from build123d import *

# Parameters (mm, degrees)
F1_DEPTH = 3
F3_DEPTH = 3


with BuildPart() as f1:
    # F0 (on Right) → F1 (new body)
    with BuildSketch(Plane.YZ):
        with BuildLine():
            ThreePointArc((0, -35), (-35, 0), (0, 35))
            Line((0, 35), (0, 50))
            Line((0, 50), (-22, 50))
            ThreePointArc((-22, 50), (-29.119444, 48.689931), (-35.306192, 44.931351))
            Line((-35.306192, 44.931351), (-125, -35))
            Line((-125, -35), (-125, -100))
            Line((-125, -100), (-105, -100))
            Line((-105, -100), (0, -50))
            Line((0, -50), (0, -35))
        make_face()
        with BuildLine():
            ThreePointArc((-96.275498, -75.908841), (-103.504138, -75.479065), (-107, -69.137387))
            Line((-107, -69.137387), (-107, -46.431792))
            ThreePointArc((-107, -46.431792), (-106.343744, -43.363703), (-104.489822, -40.832535))
            Line((-104.489822, -40.832535), (-65.699873, -6.264563))
            ThreePointArc((-65.699873, -6.264563), (-57.267065, -4.57705), (-51.677673, -11.113001))
            ThreePointArc((-51.677673, -11.113001), (-46.996343, -24.335108), (-38.322833, -35.358229))
            ThreePointArc((-38.322833, -35.358229), (-36.281412, -38.203278), (-35.560135, -41.629861))
            ThreePointArc((-35.560135, -41.629861), (-36.8729, -46.167883), (-40.405699, -49.304175))
            Line((-40.405699, -49.304175), (-96.275498, -75.908841))
        make_face(mode=Mode.SUBTRACT)
    extrude(amount=F1_DEPTH)

    # F2 (on Right) → F3 (join)
    with BuildSketch(Plane.YZ):
        with BuildLine():
            ThreePointArc((0, -35), (-35, 0), (0, 35))
            Line((0, 35), (0, 50))
            Line((0, 50), (-18.720067, 50))
            ThreePointArc((-18.720067, 50), (-21.972131, 49.787579), (-25.168931, 49.153926))
            Line((-25.168931, 49.153926), (-125, 22.5))
            Line((-125, 22.5), (-125, -22.5))
            Line((-125, -22.5), (-25.168931, -49.153926))
            ThreePointArc((-25.168931, -49.153926), (-21.972131, -49.787579), (-18.720067, -50))
            Line((-18.720067, -50), (0, -50))
            Line((0, -50), (0, -35))
        make_face()
        with BuildLine():
            Line((-103.289773, 9.665908), (-56.184511, 22.242556))
            ThreePointArc((-56.184511, 22.242556), (-51.209908, 20.791419), (-50.193177, 15.710206))
            ThreePointArc((-50.193177, 15.710206), (-52.998976, 0.017361), (-50.400586, -15.711156))
            ThreePointArc((-50.400586, -15.711156), (-51.461758, -20.754404), (-56.413973, -22.181292))
            Line((-56.413973, -22.181292), (-103.289773, -9.665908))
            ThreePointArc((-103.289773, -9.665908), (-105.965404, -7.880705), (-107, -4.835123))
            Line((-107, -4.835123), (-107, 4.835123))
            ThreePointArc((-107, 4.835123), (-105.965404, 7.880705), (-103.289773, 9.665908))
        make_face(mode=Mode.SUBTRACT)
    extrude(amount=F3_DEPTH)


solid = f1.part
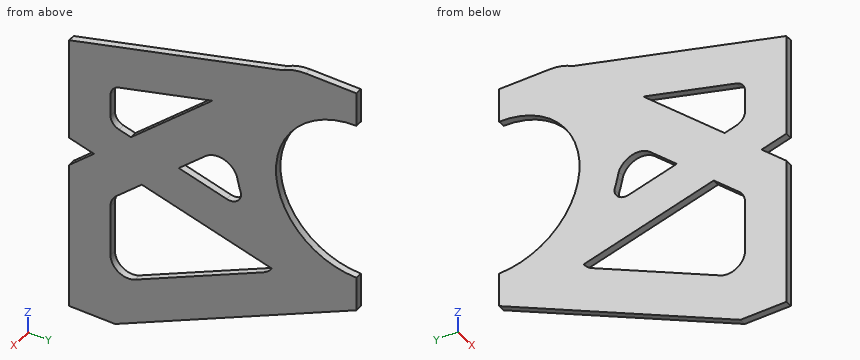
CAD build for the part. Positions are in the model's coordinates, mm. Coordinates: 2 decimals unless noted, no trailing zeros. Loops run counter-clockwise (first coordinate to the right, second up) from the corner with the lowest first, then second, coordinate; pieces in that order, holes last. Notation, with made-up numbers: (50.25, -30) -> (93.25, -30) arc R8 cw to (93.25, -23) -> close; hole circle Ø8 at (18, 50.25). An arc over 180 degrees is marked (long way). One line per item, written item: value.
1. Slice it at B-B on z = -57.5. Write the cut outline in (x, y).
Answers:
outline: (0, -125) -> (3, -125) -> (3, -107) -> (0, -107) -> close; (0, -57.62) -> (3, -57.62) -> (3, -15.75) -> (0, -15.75) -> close
2. Slice it at A-A on y = -27. Write the cut outline in (x, z).
Answers:
outline: (0, -62.86) -> (3, -62.86) -> (3, -22.27) -> (0, -22.27) -> close; (0, 22.27) -> (3, 22.27) -> (3, 49.36) -> (0, 49.36) -> close
3. Slice it at C-C on x = 0.75. Give the number of separate pieces and of enclosed holes in the cut face, and give its area (3 significant figures).
Answers:
separate pieces: 1
enclosed holes: 3
area: 10,100 mm^2
4. Drill centre lines: line 1 (Z direction, x = 0.45, y = -96); line 2 (Z direction, x = 1.25, y = -66); line 3 (Z direction, x = 0.75, y = -101.5). Where is each one in solid material? Low to high. Write a range as [from, to].
Answers:
line 1: z = [-95.71, -75.78], [-33.27, -9.16], [11.61, 30.24]
line 2: z = [-81.43, -61.49], [-38.25, -19.62], [-6.53, 17.58], [19.62, 38.25]
line 3: z = [-98.33, -76.37], [-38.17, -10.14], [10.14, 28.77]
5. Flat gauge pins, fed straight in: P1, Ø1.5, axis at x = 2.5, y = -33.5, coming from the -Z side; P2, Ø1.5, axis at x = 2, z = -52.5, coming from the +Y side (3 decimals). Where does each tip first touch, or does it go through?
Answers:
P1: stops at z = -66.31
P2: stops at y = -3.675
